from build123d import *

# Parameters (mm, degrees)
BOSS_EXTRUDE1_DEPTH      = 28.575
HOLE1_D                  = 6.35
HOLE1_DEPTH              = 6.35
HOLE1_CBORE_D            = 12.7
HOLE1_CBORE_DEPTH        = 3.175
HOLE1_TIP                = 1.907732465
F_5_16_18_TAPPED_HOLE1_D = 6.5278


with BuildPart() as part:
    # Sketch1 → Boss-Extrude1 (new body)
    with BuildSketch(Plane(origin=(0, 0, 0), x_dir=(1, 0, 0), z_dir=(0, 1, 0))):
        Polygon((-52.3875, 0), (52.3875, 0), (52.3875, -12.7), (28.575, -12.7), (28.575, -6.35), (-28.575, -6.35), (-28.575, -12.7), (-52.3875, -12.7), align=None)
    extrude(amount=BOSS_EXTRUDE1_DEPTH)

    # Hole1
    with Locations(Plane(origin=(0, 0, 6.35), x_dir=(-1, 0, 0), z_dir=(0, 0, 1))):
        with Locations((-12.7, -14.2875), (12.7, -14.2875)):
            CounterBoreHole(HOLE1_D / 2, HOLE1_CBORE_D / 2, HOLE1_CBORE_DEPTH, depth=HOLE1_DEPTH)
            with Locations((0, 0, -(HOLE1_DEPTH + HOLE1_TIP / 2))):  # 118° drill point
                Cone(0, HOLE1_D / 2, HOLE1_TIP, mode=Mode.SUBTRACT)

    # 5/16-18 Tapped Hole1 (through all)
    with Locations(Plane.XY.offset(12.7)):
        with Locations((-39.6875, 14.2875), (39.6875, 14.2875)):
            Hole(F_5_16_18_TAPPED_HOLE1_D / 2)


solid = part.part
Here's how the part is built. I have some questions about the finished solid (model axes, mm). A direction names the side the tool comes from. Round coordinates to 2 decimals unless told otherwise and drop trailing zeros. Write each loop counter-clockwise with the first axis right and the second up, starting at its lowest first coordinate (ties: lowest second). Pieces come first, ordered by that corner, then holes. Notation, with made-up numbers: (32.5, 2) -> (65.5, 2) arc R20 cw to (65.5, 9) -> close; hole circle Ø7 at (72, -15). An arc over 180 degrees is marked (long way). One line per item, written item: value.
1) I'm going to push flat-ended pins straight in: pin 1 Ø6.5 at (x, y) = (-10, 15) entering from +Z (3 decimals); pin 2 Ø8.5 at (x, y) = (-5, 11) entering from +Z. Where does each tip first touch, or does it pass through?
Filled sheet:
pin 1: stops at z = 3.175
pin 2: stops at z = 6.35
2) If I drill on line 1 (X direction, y = 14.5, z = 10.75) (1 decimal); line 2 (X direction, y = 22.75, z = 9.5) (1 decimal); line 3 (Y direction, x = -12.7, z = 1) (1 decimal), over which ranges is the centre line in solid material (lowest first)? Write a range as [from, to].
Filled sheet:
line 1: x = [-52.4, -42.9], [-36.4, -28.6], [28.6, 36.4], [42.9, 52.4]
line 2: x = [-52.4, -28.6], [28.6, 52.4]
line 3: y = [0, 11.1], [17.5, 28.6]
3) Suppose I cut it at C-C on y = 15.25. Give the number of separate pieces and of enclosed holes in the cut face, plus the area to 3 significant figures.
Filled sheet:
separate pieces: 5
enclosed holes: 0
area: 691 mm2
4) We'd pull the mould along Y, two halves only. Please class faces 4 (the face through (-13.11, 11.14, 1.57)), 5 (the face through (0, 14, 6.35)), 6 (the face through (1, 28.575, 5)): released by +Y, released by -Y, zero draft, split by the parting line, or undercut.
Filled sheet:
face 4: undercut
face 5: zero draft
face 6: released by +Y
5) For faces 1 (the face through (6.643, 12.38, 4.785)), 2 (the face through (-41.44, 17.04, 6.26)), 3 (the face through (-28.575, 14, 9)), which set-ups out of +Z, -Z, +X, -X, +Y, -Y let a thin tool reach every point of the face, with its end or its side?
Filled sheet:
face 1: +Z
face 2: +Z, -Z
face 3: +Z, +Y, -Y
6) Suppose I cut it at B-B on z = 9.75. List the corners of the cut face in (x, y) for me (1 decimal).
Filled sheet:
outline: (-52.4, 0) -> (-28.6, 0) -> (-28.6, 28.6) -> (-52.4, 28.6) -> close; (28.6, 0) -> (52.4, 0) -> (52.4, 28.6) -> (28.6, 28.6) -> close; hole circle Ø6.5 at (-39.7, 14.3); hole circle Ø6.5 at (39.7, 14.3)
